```python
from build123d import *

# Parameters (mm, degrees)
SKETCH1_W           = 56
SKETCH1_H           = 26
SKETCH1_W_2         = 24
SKETCH1_H_2         = 9
BOSS_EXTRUDE1_DEPTH = 7
SKETCH2_R           = 1.25
CUT_EXTRUDE1_DEPTH  = 7
SKETCH3_R           = 2.65
CUT_EXTRUDE2_DEPTH  = 4.6
SKETCH4_W           = 7
SKETCH4_H           = 26
BOSS_EXTRUDE2_DEPTH = 15


with BuildPart() as part:
    # Sketch1 → Boss-Extrude1 (new body)
    with BuildSketch(Plane.XY):
        Rectangle(SKETCH1_W, SKETCH1_H)
        with Locations((-5, 17.5)):
            Rectangle(SKETCH1_W_2, SKETCH1_H_2)
    extrude(amount=BOSS_EXTRUDE1_DEPTH)

    # Sketch2 → Cut-Extrude1 (cut)
    with BuildSketch(Plane.XY.offset(7)):
        with Locations((-5, 17.5)):
            Circle(SKETCH2_R)
        with Locations((-23, -0.5)):
            Circle(SKETCH2_R)
    extrude(amount=-CUT_EXTRUDE1_DEPTH, mode=Mode.SUBTRACT)

    # Sketch3 → Cut-Extrude2 (cut)
    with BuildSketch(Plane(origin=(0, 0, 0), x_dir=(-1, 0, 0), z_dir=(0, 0, -1))):
        with Locations((-5.25, 7.25)):
            Circle(SKETCH3_R)
        with Locations((-19.25, 7.25)):
            Circle(SKETCH3_R)
    extrude(amount=-CUT_EXTRUDE2_DEPTH, mode=Mode.SUBTRACT)

    # Sketch4 → Boss-Extrude2 (add)
    with BuildSketch(Plane(origin=(28, 0, 0), x_dir=(0, 0, -1), z_dir=(1, 0, 0))):
        with Locations((-3.5, 0)):
            Rectangle(SKETCH4_W, SKETCH4_H)
    extrude(amount=BOSS_EXTRUDE2_DEPTH)


solid = part.part
```
Work out the finished part from the listing and answer in its coordinate system (mm). A direction names the side the tool comes from. Give positions to 0.01 mm unless a question says otherwise; leave off trailing zeros. Loops run counter-clockwise (first coordinate to the right, second up) from the corner with the lowest first, then second, coordinate; pieces in that order, holes last. Notation, with made-up numbers: (82.25, 65) -> (119.25, 65) arc R18 cw to (119.25, 94) -> close; hole circle Ø3 at (59.25, -26.75). An arc over 180 degrees is marked (long way). Put each result on its own line as item: value. Start each with the question number.
Item 1: The part is cut by section C-C (x = 5.25). Give the vertices of the cut face in (y, z), then the cut area to 3 significant figures.
Item 2: Each of these flat-tipped pins is pushed along its axis until it touches: P1, Ø3.5, axis at x = 27.5, z = 3, coming from the +Y side; P2, Ø3.5, axis at y = 16.5, z = 2, coming from the -X side; P3, Ø1.6, axis at x = 6, y = 7.5, coming from the -Z side. Where does it stop, or does it pass through?
Item 3: The part is cut by section D-D (z = 1.5). Give the vertices of the cut face in (x, y), then the cut area to 3 significant figures.
Item 4: The mould has two halves that part along X. Classify faces 6 (the face through (16.8, 6.24, 2.27)), 7 (the face through (-17, 17, 3)), 8 (the face through (-5, 22, 3)), 9 (the face through (43, 0, 4)): released by +X, released by -X, zero draft, split by the parting line, or undercut.
Item 5: Which of the six approach directions +Z, -Z, +X, -X, +Y, -Y give full straight-line access (tool end or side, diameter ignored) to faces 1 (the face through (-5.921, 18.345, 3.549)), 2 (the face through (-23, 13, 3)), 3 (the face through (5.82, 4.66, 2.27)), 4 (the face through (-28, 0, 3)), 5 (the face through (25, 13, 4))?
Item 6: Find the intervals of material crossed by L1, parallel to Y at x = 19.25, z = 3.3; L2, parallel to Y at x = -23, z = 2.25; L3, parallel to Y at x = 30.5, z = 0.5, in increasing order. Write a range as [from, to].
Item 7: The part is cut by section B-B (y = 17.5). Give the vertices of the cut face in (x, z).
Item 8: The part is cut by section A-A (z = 6). Give the vertices of the cut face in (x, y), then the cut area to 3 significant figures.
Answers below:
1. outline: (-13, 0) -> (4.6, 0) -> (4.6, 4.6) -> (9.9, 4.6) -> (9.9, 0) -> (22, 0) -> (22, 7) -> (-13, 7) -> close
1. area: 221 mm2
2. P1: y = 13
2. P2: x = -17
2. P3: z = 4.6
3. outline: (-28, -13) -> (43, -13) -> (43, 13) -> (7, 13) -> (7, 22) -> (-17, 22) -> (-17, 13) -> (-28, 13) -> close; hole circle Ø2.5 at (-23, -0.5); hole circle Ø2.5 at (-5, 17.5); hole circle Ø5.3 at (5.25, 7.25); hole circle Ø5.3 at (19.25, 7.25)
3. area: 2,010 mm2
4. face 6: undercut
4. face 7: released by -X
4. face 8: zero draft
4. face 9: released by +X
5. face 1: +Z, -Z
5. face 2: +Z, -Z, -X, +Y
5. face 3: -Z
5. face 4: +Z, -Z, -X, +Y, -Y
5. face 5: +Z, -Z, +X, +Y
6. L1: [-13, 4.6], [9.9, 13]
6. L2: [-13, -1.75], [0.75, 13]
6. L3: [-13, 13]
7. outline: (-17, 0) -> (-6.25, 0) -> (-6.25, 7) -> (-17, 7) -> close; (-3.75, 0) -> (7, 0) -> (7, 7) -> (-3.75, 7) -> close
8. outline: (-28, -13) -> (43, -13) -> (43, 13) -> (7, 13) -> (7, 22) -> (-17, 22) -> (-17, 13) -> (-28, 13) -> close; hole circle Ø2.5 at (-23, -0.5); hole circle Ø2.5 at (-5, 17.5)
8. area: 2,050 mm2
